```python
from build123d import *

# Parameters (mm, degrees)
SKETCH1_W           = 80
SKETCH1_H           = 50
BOSS_EXTRUDE1_DEPTH = 0.4
SKETCH2_W           = 80
SKETCH2_H           = 50
SKETCH2_W_2         = 76
SKETCH2_H_2         = 46
BOSS_EXTRUDE2_DEPTH = 20
SKETCH3_W           = 70
SKETCH3_H           = 40
CUT_EXTRUDE1_DEPTH  = 98.729539691


with BuildPart() as part:
    # Sketch1 → Boss-Extrude1 (new body)
    with BuildSketch(Plane(origin=(0, 0, 0), x_dir=(1, 0, 0), z_dir=(0, 1, 0))):
        with Locations((40.973770478, -25.775500222)):
            Rectangle(SKETCH1_W, SKETCH1_H)
    extrude(amount=BOSS_EXTRUDE1_DEPTH)

    # Sketch2 → Boss-Extrude2 (add)
    with BuildSketch(Plane(origin=(0, 0.4, 0), x_dir=(1, 0, 0), z_dir=(0, 1, 0))):
        with Locations((40.973770478, -25.775500222)):
            Rectangle(SKETCH2_W, SKETCH2_H)
        with Locations((40.973770478, -25.775500222)):
            Rectangle(SKETCH2_W_2, SKETCH2_H_2, mode=Mode.SUBTRACT)
    extrude(amount=BOSS_EXTRUDE2_DEPTH)

    # Sketch3 → Cut-Extrude1 (cut, through all)
    with BuildSketch(Plane(origin=(0, 0, 0), x_dir=(-1, 0, 0), z_dir=(0, -1, 0))):
        with Locations((-40.973770478, -25.775500222)):
            Rectangle(SKETCH3_W, SKETCH3_H)
    extrude(amount=-CUT_EXTRUDE1_DEPTH, mode=Mode.SUBTRACT)


solid = part.part
```
Geometry: final body of the model. Coordinates: model frame, mm. A direction names the side the tool comes from. Give positions to 0.01 mm unless a question says otherwise; leave off trailing zeros. Write each loop counter-clockwise with the first axis right and the second up, starting at its lowest first coordinate (ties: lowest second). Pieces come first, ordered by that corner, then holes.
1. Section query C-C, the plane z = 16.5. Return loops of the section in (x, y).
2. Line query: probe 1 along X at (y, z) = (2, 45); probe 2 along Z at (x, y) = (9.5, 19); probe 3 along Y at (x, z) = (78.5, 35.5). Output: solid intervals per line, ascending.
3. Section query B-B, the plane y = 10.75. Return loops of the section in (x, z), then the cut area to 3 significant figures.
4. Draft query along Z for faces 1 (the flat face through (2.974, 10, 26)), 2 (the flat face through (40, 10, 0.776)), 3 (the flat face through (38, 20.4, 50)). Return one class per face: released by +Z, released by -Z, zero draft, split by the parting line, or undercut.
5. Section query A-A, the plane x = 36. Return loops of the section in (y, z).
6. Reachability of faces 4 (the flat face through (40, 10, 50.776)), 5 (the flat face through (40, 10, 2.776)) from +Z, -Z, +X, -X, +Y, -Y: full face, straight path, thin tool, end or side. Return the list, or none.
Computed:
1. outline: (0.97, 0) - (5.97, 0) - (5.97, 0.4) - (2.97, 0.4) - (2.97, 20.4) - (0.97, 20.4) - close; (75.97, 0) - (80.97, 0) - (80.97, 20.4) - (78.97, 20.4) - (78.97, 0.4) - (75.97, 0.4) - close
2. probe 1: x = 0.97 to 2.97, 78.97 to 80.97
2. probe 2: z = 0.78 to 2.78, 48.78 to 50.78
2. probe 3: y = 0 to 0.4
3. outline: (0.97, 0.78) - (80.97, 0.78) - (80.97, 50.78) - (0.97, 50.78) - close; hole (2.97, 2.78) - (78.97, 2.78) - (78.97, 48.78) - (2.97, 48.78) - close
3. area: 504 mm2
4. face 1: undercut
4. face 2: released by -Z
4. face 3: zero draft
5. outline: (0, 0.78) - (20.4, 0.78) - (20.4, 2.78) - (0.4, 2.78) - (0.4, 5.78) - (0, 5.78) - close; (0, 45.78) - (0.4, 45.78) - (0.4, 48.78) - (20.4, 48.78) - (20.4, 50.78) - (0, 50.78) - close
6. face 4: +Z, +X, -X, +Y, -Y
6. face 5: +Y
